Here's the drawing with two shaded views (mm, measured from the low corner). I have some questions. A direction names the side the tool comes from. Coordinates: 2 decimals unless noted, no trailing zeros. Write each loop counter-clockwise with the first axis right and the second up, starting at its lowest first coordinate (ties: lowest second). Pieces come first, ordered by that corner, then holes.
Item 1: If I drill on line 1 (Y direction, x = 11.5, z = 1.45); line 2 (Y direction, x = 24, z = 42), over which ranges is the centre line in solid material (lowest first)?
Item 2: If we section it at D-D (z = 46.5): Please give me the cut outline in (x, y), then the cut area to 3 significant figures.
Item 3: If we section it at A-A (x = 11.5): Please give me the cut outline in (y, z).
Item 4: If we section it at C-C (x = 26): Please give me the cut outline in (y, z).
Item 5: If we section it at B-B (y = 28): Please give me the cut outline in (x, z), then the cut area to 3 significant figures.
Item 6: I'm going to push flat-ended pins straight in: pin 1 Ø8 at (x, y) = (27.5, 42) entering from +Z; pin 2 Ø8 at (x, z) = (14, 46) entering from +Y. Where does each tip first touch, or does it pass through?
Item 7: For the marked faces 1 and 2, which set-ups out of +Z, -Z, +X, -X, +Y, -Y let a thin tool reach every point of the face, with its end or its side?
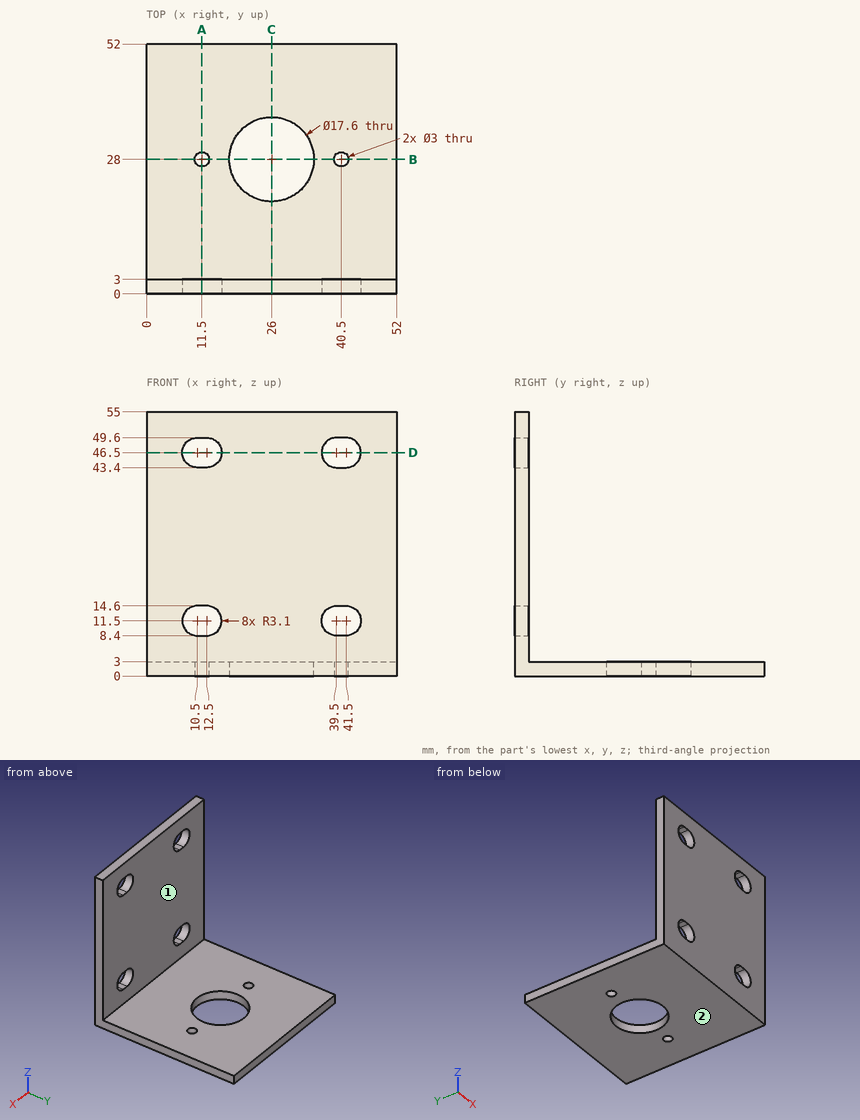
Answer list:
1. line 1: y = 0 to 26.5, 29.5 to 52
1. line 2: y = 0 to 3
2. outline: (0, 0) - (7.4, 0) - (7.4, 3) - (0, 3) - close; (15.6, 0) - (36.4, 0) - (36.4, 3) - (15.6, 3) - close; (44.6, 0) - (52, 0) - (52, 3) - (44.6, 3) - close
2. area: 107 mm2
3. outline: (0, 0) - (26.5, 0) - (26.5, 3) - (3, 3) - (3, 8.4) - (0, 8.4) - close; (0, 14.6) - (3, 14.6) - (3, 43.4) - (0, 43.4) - close; (0, 49.6) - (3, 49.6) - (3, 55) - (0, 55) - close; (29.5, 0) - (52, 0) - (52, 3) - (29.5, 3) - close
4. outline: (0, 0) - (19.2, 0) - (19.2, 3) - (3, 3) - (3, 55) - (0, 55) - close; (36.8, 0) - (52, 0) - (52, 3) - (36.8, 3) - close
5. outline: (0, 0) - (10, 0) - (10, 3) - (0, 3) - close; (13, 0) - (17.2, 0) - (17.2, 3) - (13, 3) - close; (34.8, 0) - (39, 0) - (39, 3) - (34.8, 3) - close; (42, 0) - (52, 0) - (52, 3) - (42, 3) - close
5. area: 85.2 mm2
6. pin 1: stops at z = 3
6. pin 2: stops at y = 3
7. face 1: +Z, +X, -X, +Y
7. face 2: -Z, +X, -X, +Y, -Y
